Geometry check sheet. Reference: the model listing, model coordinates, mm. A direction names the side the tool comes from. Coordinates: 2 decimals unless noted, no trailing zeros. Order: outer loops, then holes, each group sorted by start corner. A loop starts at its lowest first (then second) coordinate and runs counter-clockwise, first axis right, second up. Notation, with made-up numbers: (78, 33) - (127, 33) arc R23 cw to (127, 65) - close; hole circle Ø11 at (5, -36.75). An arc over 180 degrees is marked (long way). Put each result on its own line as item: value.
from build123d import *

# Parameters (mm, degrees)
F0_W     = 221.675306
F0_H     = 202.127948
F0_R     = 9.121421
F0_R_2   = 8.929781
F0_R_3   = 8.997318
F0_R_4   = 9.484007
F1_DEPTH = 9.525
F2_W     = 48.670978
F2_H     = 202.127948
F3_DEPTH = 38.1
F5_D     = 25.4
F6_R     = 24.13


with BuildPart() as f1:
    # F0 (on Top) → F1 (new body)
    with BuildSketch(Plane.XY):
        Rectangle(F0_W, F0_H)
        with Locations((-85.051782, -78.605309)):
            Circle(F0_R, mode=Mode.SUBTRACT)
        with Locations((87.547183, -78.605309)):
            Circle(F0_R_2, mode=Mode.SUBTRACT)
        with Locations((-85.051782, 80.268927)):
            Circle(F0_R_3, mode=Mode.SUBTRACT)
        with Locations((87.547183, 80.268927)):
            Circle(F0_R_4, mode=Mode.SUBTRACT)
    extrude(amount=F1_DEPTH)

    # F2 (on face) → F3 (join)
    with BuildSketch(Plane.XY.offset(9.525)):
        Rectangle(F2_W, F2_H)
    extrude(amount=F3_DEPTH)

    # F5 (through all)
    with Locations(Plane.XZ.offset(101.063974)):
        with Locations((0, 30.051572)):
            Hole(F5_D / 2)

    # F6
    f6_edges = [f1.edges().sort_by_distance(p)[0] for p in [
        (-24.335489, 0, 47.625),
        (24.335489, 0, 47.625),
    ]]
    fillet(f6_edges, radius=F6_R)


solid = f1.part
Q1. Section check B-B on y = 85. Record the boundary of the cut face in (x, z) (1 decimal), then the cut area to 3 significant figures.
Answer block:
outline: (-110.8, 0) - (-92.7, 0) - (-92.7, 9.5) - (-110.8, 9.5) - close; (-77.4, 0) - (79.3, 0) - (79.3, 9.5) - (24.3, 9.5) - (24.3, 23.5) arc R24.1 ccw to (0.2, 47.6) - (-0.2, 47.6) arc R24.1 ccw to (-24.3, 23.5) - (-24.3, 9.5) - (-77.4, 9.5) - close; (95.8, 0) - (110.8, 0) - (110.8, 9.5) - (95.8, 9.5) - close; hole circle Ø25.4 at (0, 30.1)
area: 2,910 mm^2
Q2. Section check C-C on z = 4. Record the boundary of the cut face in (x, y), then the cut area to 3 significant figures.
Answer block:
outline: (-110.84, -101.06) - (110.84, -101.06) - (110.84, 101.06) - (-110.84, 101.06) - close; hole circle Ø18.24 at (-85.05, -78.61); hole circle Ø17.99 at (-85.05, 80.27); hole circle Ø18.97 at (87.55, 80.27); hole circle Ø17.86 at (87.55, -78.61)
area: 43,800 mm^2
Q3. Section check D-D on y = 64.5. Record the boundary of the cut face in (x, z) (3 decimals).
Answer block:
outline: (-110.838, 0) - (110.838, 0) - (110.838, 9.525) - (24.335, 9.525) - (24.335, 23.495) arc R24.13 ccw to (0.205, 47.625) - (-0.205, 47.625) arc R24.13 ccw to (-24.335, 23.495) - (-24.335, 9.525) - (-110.838, 9.525) - close; hole circle Ø25.4 at (0, 30.052)
Q4. Depth check by flat-ended pin: pin 1 Ø12 at (x, y) = (29.5, -6) entering from -Z; pin 2 Ø1 at (y, z) = (-33.5, 22) entering from -X; pin 3 Ø1 at (x, y) = (64.5, -49.5) entering from +Z (3 decimals); pin 4 Ø1.5 at (x, y) = (15, -1) entering from +Z. Enter the tip coordinate at first touch or a pass-through.
Answer block:
pin 1: stops at z = 0
pin 2: stops at x = -24.34
pin 3: stops at z = 9.525
pin 4: stops at z = 43.12
Q5. Thickness scan on L1, parallel to Z at x = 0, y = 60 (3 decimals); L2, parallel to Z at x = -34, y = -1.5 (3 decimals); L3, parallel to X at y = -5, z = 16. Record the ranges inside material, lowest first. Write a range as [from, to].
Answer block:
L1: z = [0, 17.352], [42.752, 47.625]
L2: z = [0, 9.525]
L3: x = [-24.34, 24.34]
Q6. Section check A-A on z = 34. Record the boundary of the cut face in (x, y).
Answer block:
outline: (-21.93, -101.06) - (-12.07, -101.06) - (-12.07, 101.06) - (-21.93, 101.06) - close; (12.07, -101.06) - (21.93, -101.06) - (21.93, 101.06) - (12.07, 101.06) - close
Q7. Draft check along Y on faces 1 (the cylindrical face through (-80.215, 87.856, 4.696)), 2 (the flat face through (-1, 101.064, 11)), 3 (the flat face through (110.838, -1, 5)), 4 (the cylindrical face through (80.56, 86.68, 4.7)). Enter one of: pulls with the +Y half, pulls with the -Y half, needs draft (parallel to the pull), parting line crosses it, or undercut.
Answer block:
face 1: undercut
face 2: pulls with the +Y half
face 3: needs draft
face 4: undercut
Q8. Access from +Z, -Z, +X, -X, +Y, -Y to the whole of each face (thin tool, end or side, straight path). Record for faces 5 (the flat face through (24.335, -1, 16)), 6 (the flat face through (-110.838, -1, 5)), 7 (the flat face through (-24.335, -1, 16)).
Answer block:
face 5: +Z, +X, +Y, -Y
face 6: +Z, -Z, -X, +Y, -Y
face 7: +Z, -X, +Y, -Y
